For this review, use the dimensioned drawing (mm, ordinates from the lowest corner) and the shaded views. A direction names the side the tool comes from. Coordinates: 2 decimals unless noted, no trailing zeros. Write each loop counter-clockwise with the first axis right and the second up, starting at its lowest first coordinate (ties: lowest second). Pieces come first, ordered by that corner, then holes. Notation, with made-up numbers: (80, 10.25) - (117, 10.25) arc R20 ccw to (117, 46.25) - close; hole circle Ø10 at (57, 31.5). An arc over 180 degrees is marked (long way). Put each result on its own line as item: value.
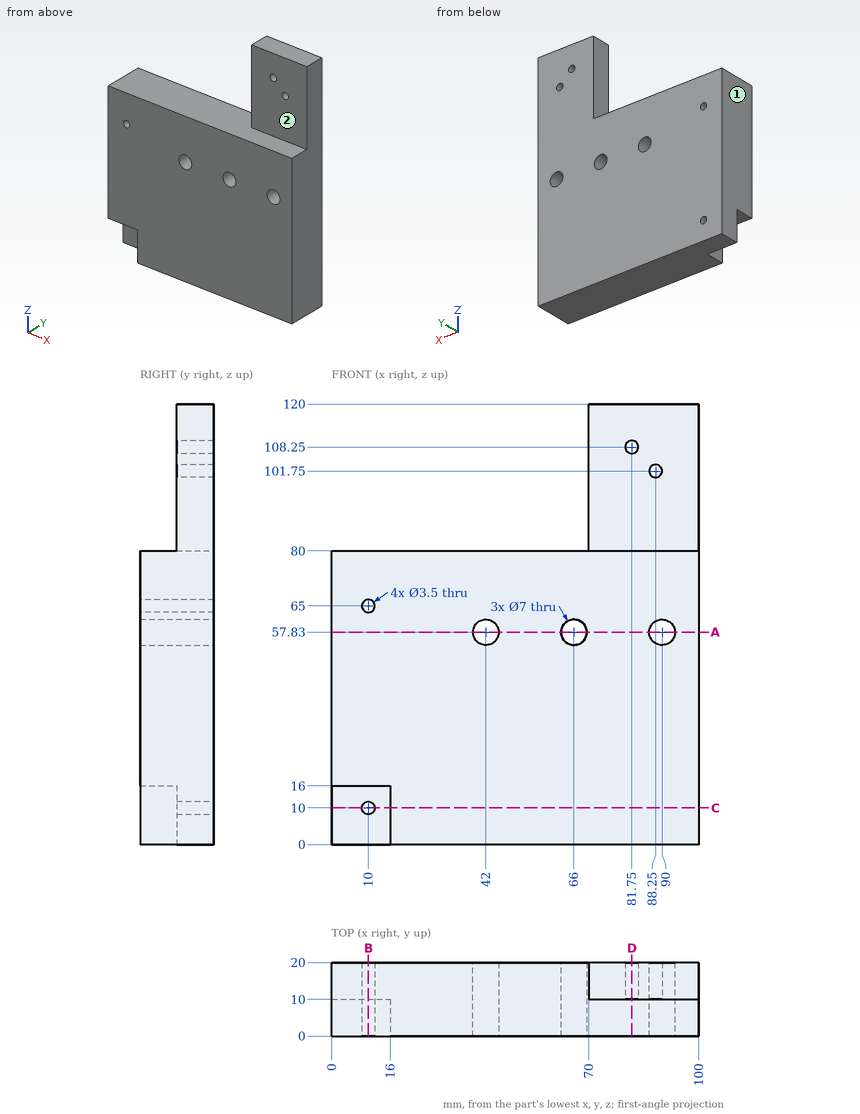
1. To check wall thickness, follow probe 1 along X at (y, z) = (8.75, 57.83); probe 2 along Z at (x, y) = (10, 16.75); probe 3 along X at (y, z) = (13.5, 10). State the ranges of each line that lie inside material, in increasing order.
Determined:
probe 1: x = 0 to 38.5, 45.5 to 62.5, 69.5 to 86.5, 93.5 to 100
probe 2: z = 0 to 8.25, 11.75 to 63.25, 66.75 to 80
probe 3: x = 0 to 8.25, 11.75 to 100
2. For pin 1 Ø3 at (x, y) = (4.5, 2.5) entering from -Z; pin 2 Ø8 at (y, z) = (11, 91) entering from -X; pin 3 Ø8 at (y, z) = (2.5, 11) entering from -X; pin 4 Ø24 at (x, z) = (80.5, 90) entering from -Y, all flat-tipped, find the tip position at first contact; note any pin that passes through.
Determined:
pin 1: stops at z = 16
pin 2: stops at x = 70
pin 3: stops at x = 16
pin 4: stops at y = 0
3. Consider section B-B on x = 10. State the section outline as (y, z) points, plus the area to 4 significant figures.
Determined:
outline: (0, 16) - (10, 16) - (10, 11.75) - (20, 11.75) - (20, 63.25) - (0, 63.25) - close; (0, 66.75) - (20, 66.75) - (20, 80) - (0, 80) - close; (10, 0) - (20, 0) - (20, 8.25) - (10, 8.25) - close
area: 1,335 mm^2
4. Consider section D-D on x = 81.75. State the section outline as (y, z) points.
Determined:
outline: (0, 0) - (20, 0) - (20, 106.5) - (10, 106.5) - (10, 80) - (0, 80) - close; (10, 110) - (20, 110) - (20, 120) - (10, 120) - close
5. Machinability: for the marked faces 1 and 2, which of the approach directions +Z, -Z, +X, -X, +Y, -Y give a long, thin tool a straight path to every point of the face, cutting with its end or side? Answer none if there is none.
Determined:
face 1: +Z, -Z, -X, +Y, -Y
face 2: +Z, +X, -X, -Y
6. Consider section A-A on z = 57.83. State the section outline as (x, y) points, plus the area to 3 significant figures.
Determined:
outline: (0, 0) - (38.5, 0) - (38.5, 20) - (0, 20) - close; (45.5, 0) - (62.5, 0) - (62.5, 20) - (45.5, 20) - close; (69.5, 0) - (86.5, 0) - (86.5, 20) - (69.5, 20) - close; (93.5, 0) - (100, 0) - (100, 20) - (93.5, 20) - close
area: 1,580 mm^2
7. Consider section C-C on z = 10. State the section outline as (x, y) points.
Determined:
outline: (0, 10) - (8.25, 10) - (8.25, 20) - (0, 20) - close; (11.75, 10) - (16, 10) - (16, 0) - (100, 0) - (100, 20) - (11.75, 20) - close
